Model file for the job. Use its own axes, mm. Coordinates: 2 decimals unless noted, no trailing zeros. Loops run counter-clockwise (first coordinate to the right, second up) from the corner with the lowest first, then second, coordinate; pieces in that order, holes last.
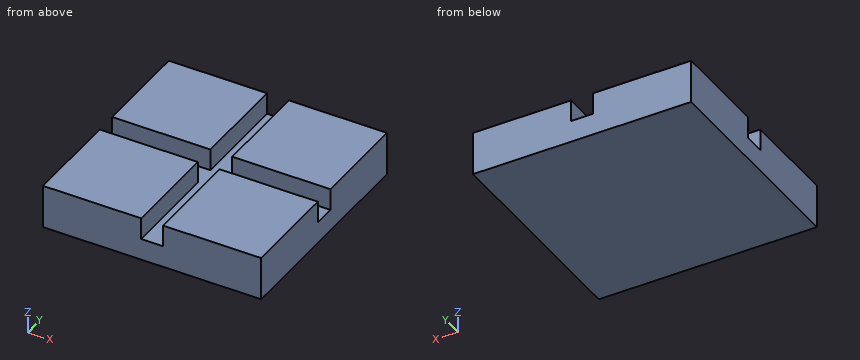
from build123d import *

# Parameters (mm, degrees)
SKETCH1_W      = 100
SKETCH1_H      = 100
EXTRUDE1_DEPTH = 20
SKETCH2_W      = 10
SKETCH2_H      = 100
EXTRUDE2_DEPTH = 10
SKETCH3_W      = 100
SKETCH3_H      = 10
EXTRUDE3_DEPTH = 10


with BuildPart() as part:
    # Sketch1 → Extrude1 (new body)
    with BuildSketch(Plane.XY):
        Rectangle(SKETCH1_W, SKETCH1_H)
    extrude(amount=-EXTRUDE1_DEPTH)

    # Sketch2 → Extrude2 (cut)
    with BuildSketch(Plane.XY):
        Rectangle(SKETCH2_W, SKETCH2_H)
    extrude(amount=-EXTRUDE2_DEPTH, mode=Mode.SUBTRACT)

    # Sketch3 → Extrude3 (cut)
    with BuildSketch(Plane.XY):
        Rectangle(SKETCH3_W, SKETCH3_H)
    extrude(amount=-EXTRUDE3_DEPTH, mode=Mode.SUBTRACT)


solid = part.part
Q1. Slice it at B-B (y = 31). List the corners of the cut face in (x, z), and give its area (3 significant figures).
Answers:
outline: (-50, -20) - (50, -20) - (50, 0) - (5, 0) - (5, -10) - (-5, -10) - (-5, 0) - (-50, 0) - close
area: 1,900 mm2
Q2. Slice it at A-A (z = -4.25). List the corners of the cut face in (x, y).
Answers:
outline: (-50, -50) - (-5, -50) - (-5, -5) - (-50, -5) - close; (-50, 5) - (-5, 5) - (-5, 50) - (-50, 50) - close; (5, -50) - (50, -50) - (50, -5) - (5, -5) - close; (5, 5) - (50, 5) - (50, 50) - (5, 50) - close
Q3. Drill centre lines: line 1 (X direction, y = -11.5, z = -1.25); line 2 (Z direction, x = 4, y = -5). Where is each one in solid material? Low to high.
Answers:
line 1: x = -50 to -5, 5 to 50
line 2: z = -20 to -10
